Autodesk Inventor part; units mm, degrees
ref_plane "YZ Plane" through (0, 0, 0) normal (1, 0, 0) x (0, 1, 0)
ref_plane "XZ Plane" through (0, 0, 0) normal (0, 1, 0) x (-1, 0, 0)
ref_plane "XY Plane" through (0, 0, 0) normal (0, 0, 1) x (1, 0, 0)
sketch "Sketch1" plane through (0, 0, 0) normal (0, 1, 0) x (-1, 0, 0)
  line L0 (-45.1427, 41.275) -> (-45.1427, -0.6244)
  arc A0 (-52.0007, -0.6244) -> (-45.1427, -0.6244) centre (-48.5717, -0.6244) ccw
  line L1 (-52.0007, -0.6244) -> (-52.0007, 41.275)
  arc A1 (-45.1427, 41.275) -> (-52.0007, 41.275) centre (-48.5717, 41.275) ccw
  arc A2 (-26.6007, -0.6244) -> (-23.1717, -4.0534) centre (-23.1717, -0.6244) ccw
  line L2 (-26.6007, -0.6244) -> (-26.6007, 50.1756)
  arc A3 (-23.1717, 53.6046) -> (-26.6007, 50.1756) centre (-23.1717, 50.1756) ccw
  arc A4 (-32.5697, 50.1756) -> (-39.1737, 50.1756) centre (-35.8717, 50.1756) ccw
  line L3 (-32.5697, 50.1756) -> (-32.5697, -0.6244)
  arc A5 (-39.1737, -0.6244) -> (-32.5697, -0.6244) centre (-35.8717, -0.6244) ccw
  line L4 (-39.1737, -0.6244) -> (-39.1737, 50.1756)
  line L5 (-23.1717, 61.3516) -> (-42.2217, 61.3516)
  arc A6 (-48.5717, 67.7016) -> (-42.2217, 61.3516) centre (-42.2217, 67.7016) ccw
  line L6 (-48.5717, 67.7016) -> (-48.5717, 122.1945)
  arc A7 (-44.852, 131.1748) -> (-48.5717, 122.1945) centre (-35.8717, 122.1945) ccw
  line L7 (-44.852, 131.1748) -> (-33.9759, 142.0509)
  arc A8 (-33.9759, 142.0509) -> (-33.046, 144.2959) centre (-36.221, 144.2959) ccw
  line L8 (-33.046, 144.2959) -> (-33.046, 154.7283)
  arc A9 (-33.046, 154.7283) -> (-34.316, 155.9983) centre (-34.316, 154.7283) ccw
  line L9 (-34.316, 155.9983) -> (-36.8109, 155.9983)
  line L10 (-61.2717, 122.3315) -> (-61.2717, -11.8004)
  line L11 (-61.2717, -11.8004) -> (-23.1717, -11.8004)
  circle A10 centre (-35.2685, 151.7756) radius 1.1303 construction
  circle A11 centre (-37.5862, 148.3847) radius 1.1303 construction
  circle A12 centre (-40.3485, 144.9938) radius 1.1303 construction
  circle A13 centre (-40.3485, 151.7756) radius 1.1303 construction
  circle A14 centre (-40.3485, 144.9938) radius 1.1303 construction
  circle A15 centre (-42.6662, 148.3847) radius 1.1303 construction
  circle A16 centre (-45.4285, 144.9938) radius 1.1303 construction
  line L12 (-34.316, 155.9983) -> (-39.3509, 155.9983)
  line L13 (-41.5959, 155.0684) -> (-55.1707, 141.4936)
  line L14 (-61.2717, 122.3315) -> (-61.2717, 131.5606)
  arc A17 (-55.1707, 141.4936) -> (-61.0225, 132.7936) centre (-35.8717, 122.1945) ccw
  arc A18 (-39.3509, 155.9983) -> (-41.5959, 155.0684) centre (-39.3509, 152.8233) ccw
  arc A19 (-61.0225, 132.7936) -> (-61.2717, 131.5606) centre (-58.0967, 131.5606) ccw
  line L15 (-23.1717, 61.3516) -> (-23.1717, 53.6046)
  line L16 (-23.1717, -4.0534) -> (-23.1717, -11.8004)
  circle A20 centre (-35.2685, 144.9938) radius 1.22
  circle A21 centre (-35.2685, 151.7756) radius 1.2192
  circle A22 centre (-37.5862, 148.3847) radius 1.2192
  circle A23 centre (-40.3485, 151.7756) radius 1.2192
  circle A24 centre (-42.6662, 148.3847) radius 1.2192
  circle A25 centre (-40.3485, 144.9938) radius 1.2192
  circle A26 centre (-45.4285, 144.9938) radius 1.2192
  line L17 (-54.9217, 50.1756) -> (-54.9217, 126.3756) construction
  circle A27 centre (-54.9217, 126.3756) radius 2.7813
  circle A28 centre (-54.9217, 50.1756) radius 2.7813
  line L18 (-61.2717, -11.8004) -> (-55.5567, -11.8004)
  line L19 (-55.5567, -11.8004) -> (-55.5567, -6.0854) construction
  line L20 (-55.5567, -6.0854) -> (-61.2717, -6.0854) construction
  line L21 (-61.2717, -6.0854) -> (-61.2717, -11.8004)
  circle A29 centre (-55.5567, -6.0854) radius 2.7813
  point P0 (-41.301, 144.2959)
  point P1 (-41.8909, 152.8233)
  point P2 (-61.2717, 132.1817)
  point P3 (-26.6007, -0.6244)
  point P4 (-32.5697, -0.6244)
  point P5 (-52.0007, -0.6244)
  point P6 (-45.1427, -0.6244)
  dimension "d2" = 3.175
  dimension "d12" = 2.44
  dimension "d13" = 2.4384
  dimension "d14" = 2.4384
  dimension "d15" = 2.4384
  dimension "d16" = 2.4384
  dimension "d17" = 2.4384
  dimension "d18" = 2.4384
  dimension "d19" = 76.2
  dimension "d20" = 5.5626
  dimension "d21" = 5.5626
  dimension "d23" = 5.715
  dimension "d24" = 5.715
  dimension "d25" = 5.5626
extrude "Extrusion3" add sketch "Sketch1" along normal blind 5
mirror "Mirror2" about plane through (23.1717, 0, 53.6046) normal (-1, 0, 0)
properties part number "twoSidedHeadplateHolder_wide_sendcutsend"
Design review of the part built by this model. Coordinates are the model's own, in mm. A direction names the side the tool comes from. Round coordinates to 2 decimals unless told otherwise and drop trailing zeros. Write each loop counter-clockwise with the first axis right and the second up, starting at its lowest first coordinate (ties: lowest second). Pieces come first, ordered by that corner, then holes.
Item 1: For faces 1 (the flat face through (-14.928, 2, 59)), 2 (the flat face through (1.201, 2, 20)), list the 3-axis set-ups (+Z, -Z, +X, -X, +Y, -Y) from which the entire face can be reached by the end or side of a thin tool; tool diameter is ignored.
Item 2: Draft analysis for pull direction X (two halves, no side actions). For faces 3 (the cylindrical face through (58.559, 2.465, 137.366)), 4 (the cylindrical face through (-12.134, 2.465, 137.488)), 5 (the cylindrical face through (55.52, 2.46, 129.09)), state which applies: released by +X, released by -X, zero draft, split by the parting line, or undercut.
Item 3: For pin 1 Ø1 at (x, y) = (14.5, 1.5) entering from +Z; pin 2 Ø1.5 at (y, z) = (2, 151) entering from +X, all flat-tipped, find the tip position at first contact; note any pin that passes through.
Item 4: Consider section C-C on x = 23. Give the boundary of the cut face in (y, z), and give its area (3 significant figures).
Item 5: Wall thickness on L1, parallel to X at y = 2.8, z = 77; L2, parallel to X at y = 0.9, z = 43; L3, parallel to Z at x = -1, y = 1.15: over which ranges is each line inside the solid? List them lowest first.
Item 6: Consider section A-A on z = 28. Give the boundary of the cut face in (x, y).
Item 7: Consider section D-D on y = 3.6. Count the separate pieces of the cut face and the enclosed holes in it, and give its area (3 significant figures).
Item 8: Consider section B-B on z = 92. Give the boundary of the cut face in (x, y), and give its area (3 significant figures).
Check values:
1. face 1: +Z, -Z, -X, +Y, -Y
1. face 2: +Y, -Y
2. face 3: released by +X
2. face 4: released by -X
2. face 5: undercut
3. pin 1: stops at z = 61.35
3. pin 2: stops at x = 46.41
4. outline: (0, -11.8) - (5, -11.8) - (5, -4.05) - (0, -4.05) - close; (0, 53.6) - (5, 53.6) - (5, 61.35) - (0, 61.35) - close
4. area: 77.5 mm2
5. L1: x = -14.93 to -2.23, 48.57 to 61.27
5. L2: x = -14.93 to -5.19, 0.74 to 7.17, 13.77 to 19.74, 26.6 to 32.57, 39.17 to 45.61, 51.54 to 61.27
5. L3: z = -11.8 to -3.83, 44.48 to 63.95, 127.64 to 149.32
6. outline: (-14.93, 0) - (-5.66, 0) - (-5.66, 5) - (-14.93, 5) - close; (1.2, 0) - (7.17, 0) - (7.17, 5) - (1.2, 5) - close; (13.77, 0) - (19.74, 0) - (19.74, 5) - (13.77, 5) - close; (26.6, 0) - (32.57, 0) - (32.57, 5) - (26.6, 5) - close; (39.17, 0) - (45.14, 0) - (45.14, 5) - (39.17, 5) - close; (52, 0) - (61.27, 0) - (61.27, 5) - (52, 5) - close
7. separate pieces: 1
7. enclosed holes: 25
7. area: 6,230 mm2
8. outline: (-14.93, 0) - (-2.23, 0) - (-2.23, 5) - (-14.93, 5) - close; (48.57, 0) - (61.27, 0) - (61.27, 5) - (48.57, 5) - close
8. area: 127 mm2
